from build123d import *


with BuildPart() as part:
    # Sketch1 → Revolve1 (revolve)
    with BuildSketch(Plane.XY, mode=Mode.PRIVATE) as revolve1_sk:
        with BuildLine():
            ThreePointArc((-4.873397172, 11.25), (0, 8.75), (4.873397172, 11.25))
            Line((4.873397172, 11.25), (6.75, 11.25))
            Line((6.75, 11.25), (6.75, 5.5))
            Line((6.75, 5.5), (7.25, 5.5))
            Line((7.25, 5.5), (7.25, 4))
            Line((7.25, 4), (-7.25, 4))
            Line((-7.25, 4), (-7.25, 5.5))
            Line((-7.25, 5.5), (-6.75, 5.5))
            Line((-6.75, 5.5), (-6.75, 11.25))
            Line((-6.75, 11.25), (-4.873397172, 11.25))
        make_face()
    revolve(revolve1_sk.sketch.rotate(Axis((-7.25, 0, 0), (1, 0, 0)), 90), axis=Axis((-7.25, 0, 0), (1, 0, 0)))


solid = part.part
Verification items for the finished model (mm, model axes). A direction names the side the tool comes from. Coordinates: 2 decimals unless noted, no trailing zeros. Order: outer loops, then holes, each group sorted by start corner. A loop starts at its lowest first (then second) coordinate and runs counter-clockwise, first axis right, second up. Notation, with made-up numbers: (-22, 17.5) -> (4, 17.5) arc R11 cw to (4, 21.5) -> close; hole circle Ø8 at (77.5, 15.25). An arc over 180 degrees is marked (long way). Put each result on its own line as item: value. Start each with the question number.
1. Access from +Z, -Z, +X, -X, +Y, -Y to the whole of each face (thin tool, end or side, straight path). Record for faces 1 (the cylindrical face through (5.82, 9.98, 5.19)), 2 (the flat face through (-6.75, 5, 3)), 3 (the cylindrical face through (7, 5.37, -1.19)).
2. Mould release check, pull along Y, two halves, no side actions. Record for faces 4 (the cylindrical face through (-7, 5.37, -1.19)), 5 (the cylindrical face through (-0.101, 3.905, -0.867)), 6 (the flat face through (-7.25, 2, 4)): released by +Y, released by -Y, zero draft, split by the parting line, or undercut.
3. Cross-section at D-D, the plane x = -3. Record the boundary of the cut face in (y, z), then the cut area to 3 significant figures.
4. Go/stop test with flat-tipped pins: pin 1 Ø4 at (y, z) = (-8.5, -9) entering from -X; pin 2 Ø6 at (y, z) = (-9, -2.5) entering from +X; pin 3 Ø8 at (x, z) = (4.5, -8.5) entering from +Y. Record where each tip stops, or that it passes through.
5. Cross-section at C-C, the plane x = -6.25. Record the boundary of the cut face in (y, z), then the cut area to 3 significant figures.
6. Material ranges on L1, parallel to X at y = 3, z = -5.5; L2, parallel to Y at x = 1, z = 0; L3, parallel to X at y = -7, z = 7, recorded low to high. Write a range as [from, to].
7. Cross-section at A-A, the plane z = 0. Record the boundary of the cut face in (x, y).
Computed:
1. face 1: +X, -X
1. face 2: -X
1. face 3: +X
2. face 4: split by the parting line
2. face 5: undercut
2. face 6: zero draft
3. outline: circle Ø19.11 at (0, 0); hole circle Ø8 at (0, 0)
3. area: 236 mm2
4. pin 1: x = -6.75
4. pin 2: x = 6.75
4. pin 3: y = 10.3
5. outline: circle Ø22.5 at (0, 0); hole circle Ø8 at (0, 0)
5. area: 347 mm2
6. L1: [-6.75, 6.75]
6. L2: [-8.83, -4], [4, 8.83]
6. L3: [-6.75, -3.53], [3.53, 6.75]
7. outline: (-7.25, -5.5) -> (-6.75, -5.5) -> (-6.75, -11.25) -> (-4.87, -11.25) arc R6 cw to (4.87, -11.25) -> (6.75, -11.25) -> (6.75, -5.5) -> (7.25, -5.5) -> (7.25, -4) -> (-7.25, -4) -> close; (-7.25, 4) -> (7.25, 4) -> (7.25, 5.5) -> (6.75, 5.5) -> (6.75, 11.25) -> (4.87, 11.25) arc R6 cw to (-4.87, 11.25) -> (-6.75, 11.25) -> (-6.75, 5.5) -> (-7.25, 5.5) -> close
